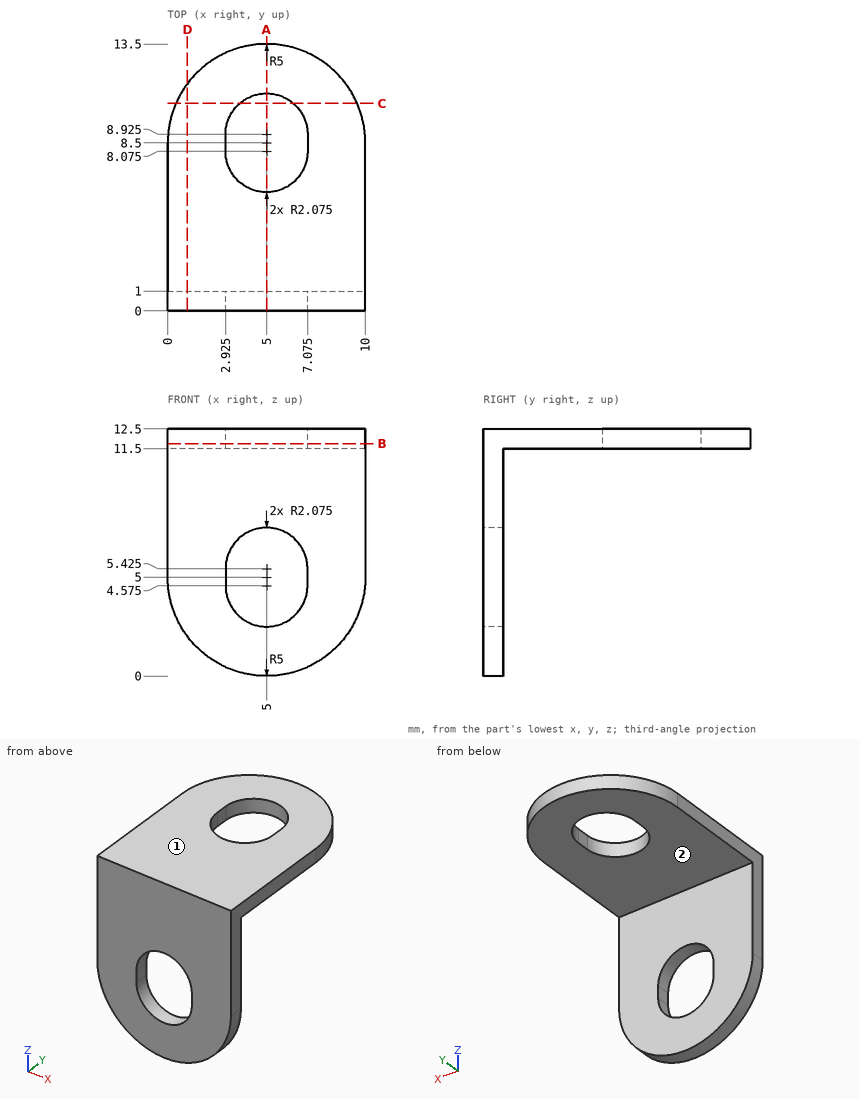
Design review of the part shown in the three views and the two pictorial views. Dimensions are in mm from the part's minimum x, y and z. A direction names the side the tool comes from. Coordinates: 2 decimals unless noted, no trailing zeros. Write each loop counter-clockwise with the first axis right and the second up, starting at its lowest first coordinate (ties: lowest second). Pieces come first, ordered by that corner, then holes.
1) We need section B-B on z = 11.75. State the section outline as (x, y) points (3 decimals).
2) We need section C-C on y = 10.5. State the section outline as (x, z) points.
3) Clearance check with flat-ended pins moving along their axes: pin 1 Ø1.5 at (x, y) = (2.5, 9.5) entering from -Z; pin 2 Ø1 at (x, y) = (5, 8) entering from -Z; pin 3 Ø1 at (x, z) = (8, 7.5) entering from +Y. State where each tip first meets the part, or that it passes through.
4) We need section A-A on x = 5. State the section outline as (y, z) points, then the cut area to 3 significant figures.
5) We need section D-D on x = 1. State the section outline as (y, z) points, then the cut area to 3 significant figures.
6) To check wall thickness, follow probe 1 along Y at (x, z) = (3.75, 1); probe 2 along X at (y, z) = (0.5, 5) (3 decimals); probe 3 along Z at (x, y) = (4.75, 4.75). State the ranges of each line that lie inside material, in increasing order.
7) Machinability: for the marked faces 1 and 2, which of the approach directions +Z, -Z, +X, -X, +Y, -Y give a long, thin tool a straight path to every point of the face, cutting with its end or side? Answer none if there is none.
Answer list:
1. outline: (0, 0) - (10, 0) - (10, 8.5) arc R5 ccw to (0, 8.5) - close; hole (2.925, 8.075) arc R2.075 ccw to (7.075, 8.075) - (7.075, 8.925) arc R2.075 ccw to (2.925, 8.925) - close
2. outline: (0.42, 11.5) - (3.65, 11.5) - (3.65, 12.5) - (0.42, 12.5) - close; (6.35, 11.5) - (9.58, 11.5) - (9.58, 12.5) - (6.35, 12.5) - close
3. pin 1: stops at z = 11.5
3. pin 2: passes through
3. pin 3: stops at y = 1
4. outline: (0, 0) - (1, 0) - (1, 2.5) - (0, 2.5) - close; (0, 7.5) - (1, 7.5) - (1, 11.5) - (6, 11.5) - (6, 12.5) - (0, 12.5) - close; (11, 11.5) - (13.5, 11.5) - (13.5, 12.5) - (11, 12.5) - close
4. area: 15.0 mm2
5. outline: (0, 2) - (1, 2) - (1, 11.5) - (11.5, 11.5) - (11.5, 12.5) - (0, 12.5) - close
5. area: 21.0 mm2
6. probe 1: y = 0 to 1
6. probe 2: x = 0 to 2.925, 7.075 to 10
6. probe 3: z = 11.5 to 12.5
7. face 1: +Z, +X, -X, +Y, -Y
7. face 2: -Z, +X, -X, +Y
